```python
from build123d import *

# Parameters (mm, degrees)
SKETCH1_W                = 2
SKETCH1_H                = 6
BOSS_EXTRUDE1_DEPTH      = 8
BOSS_EXTRUDE1_2_DEPTH    = 8
BOSS_EXTRUDE2_DEPTH      = 6
FILLET2_R                = 3
SKETCH3_R                = 1.65
CUT_EXTRUDE1_DEPTH       = 90.043007931
FILLET3_R                = 6
CIRPATTERN2_COUNT        = 3
FILLET2_OF_CIRPATTERN2_R = 3
FILLET3_OF_CIRPATTERN2_R = 6
SKETCH4_R                = 2
CUT_EXTRUDE2_DEPTH       = 80.425963387
CHAMFER1_SIZE            = 1


with BuildPart() as part:
    # Sketch1 → Boss-Extrude1 (new body)
    with BuildSketch(Plane(origin=(0, 0, 0), x_dir=(1, 0, 0), z_dir=(0, 1, 0))):
        with Locations((-24, 50)):
            Rectangle(SKETCH1_W, SKETCH1_H)
    boss_extrude1 = extrude(amount=BOSS_EXTRUDE1_DEPTH)



with BuildPart() as body_2:
    # Sketch1 → Boss-Extrude1 2 (new body)
    with BuildSketch(Plane(origin=(0, 0, 0), x_dir=(1, 0, 0), z_dir=(0, 1, 0))):
        with Locations((24, 50)):
            Rectangle(SKETCH1_W, SKETCH1_H)
    boss_extrude1_2 = extrude(amount=BOSS_EXTRUDE1_2_DEPTH)


with BuildPart() as part_1:
    add(part.part)

    add(body_2.part)  # Boss-Extrude2 merges body 2
    # Sketch2 → Boss-Extrude2 (add)
    with BuildSketch(Plane(origin=(0, 0, 0), x_dir=(1, 0, 0), z_dir=(0, 1, 0))):
        with BuildLine():
            Line((25, 53), (-25, 53))
            Line((-25, 53), (-25, 47))
            ThreePointArc((-25, 47), (-36.983431799, 38.291327639), (-46.103145229, 26.617663308))
            Line((-46.103145229, 26.617663308), (-36.806079661, 21.25))
            ThreePointArc((-36.806079661, 21.25), (0, 42.5), (36.806079661, 21.25))
            Line((36.806079661, 21.25), (46.103145229, 26.617663308))
            ThreePointArc((46.103145229, 26.617663308), (36.983431799, 38.291327639), (25, 47))
            Line((25, 47), (25, 53))
        make_face()
    boss_extrude2 = extrude(amount=-BOSS_EXTRUDE2_DEPTH)

    # Fillet2
    fillet2_edges = [part_1.edges().sort_by_distance(p)[0] for p in [
        (24, 8, -47),
        (24, 8, -53),
        (-24, 8, -47),
        (-24, 8, -53),
    ]]
    fillet(fillet2_edges, radius=FILLET2_R - 0.0001)  # a hair under: the kernel refuses the full size

    # Sketch3 → Cut-Extrude1 (cut, through all)
    with BuildSketch(Plane(origin=(25, 0, 0), x_dir=(0, 0, -1), z_dir=(1, 0, 0))):
        with Locations((50, 5)):
            Circle(SKETCH3_R)
    cut_extrude1 = extrude(amount=-CUT_EXTRUDE1_DEPTH, mode=Mode.SUBTRACT)

    # Fillet3
    fillet3_edges = [part_1.edges().sort_by_distance(p)[0] for p in [
        (0, -6, -53),
    ]]
    fillet(fillet3_edges, radius=FILLET3_R - 0.0001)  # a hair under: the kernel refuses the full size

    # CirPattern2: Boss-Extrude1, Boss-Extrude1 2, Boss-Extrude2, Cut-Extrude1 ×3 about axis
    cirpattern2_axis = Axis((0, 0, 0), (0, 1, 0))
    add([boss_extrude1.rotate(cirpattern2_axis, i * 360 / CIRPATTERN2_COUNT) for i in range(1, CIRPATTERN2_COUNT)])
    add([boss_extrude1_2.rotate(cirpattern2_axis, i * 360 / CIRPATTERN2_COUNT) for i in range(1, CIRPATTERN2_COUNT)])
    add([boss_extrude2.rotate(cirpattern2_axis, i * 360 / CIRPATTERN2_COUNT) for i in range(1, CIRPATTERN2_COUNT)])
    add([cut_extrude1.rotate(cirpattern2_axis, i * 360 / CIRPATTERN2_COUNT) for i in range(1, CIRPATTERN2_COUNT)], mode=Mode.SUBTRACT)

    # Fillet2 of CirPattern2
    fillet2_of_cirpattern2_edges = [part_1.edges().sort_by_distance(p)[0] for p in [
        (-52.703193978, 8, 2.715390309),
        (-57.899346401, 8, 5.715390309),
        (-28.703193978, 8, 44.284609691),
        (-33.899346401, 8, 47.284609691),
        (28.703193978, 8, 44.284609691),
        (33.899346401, 8, 47.284609691),
        (52.703193978, 8, 2.715390309),
        (57.899346401, 8, 5.715390309),
    ]]
    fillet(fillet2_of_cirpattern2_edges, radius=FILLET2_OF_CIRPATTERN2_R - 0.0001)  # a hair under: the kernel refuses the full size

    # Fillet3 of CirPattern2
    fillet3_of_cirpattern2_edges = [part_1.edges().sort_by_distance(p)[0] for p in [
        (-45.899346401, -6, 26.5),
        (45.899346401, -6, 26.5),
    ]]
    fillet(fillet3_of_cirpattern2_edges, radius=FILLET3_OF_CIRPATTERN2_R - 0.0001)  # a hair under: the kernel refuses the full size

    # Sketch4 → Cut-Extrude2 (cut, through all)
    with BuildSketch(Plane(origin=(0, 0, 0), x_dir=(1, 0, 0), z_dir=(0, 1, 0))):
        with Locations(Location((-41.13620668, 23.75, 0), (0, 0, 270))):
            Circle(SKETCH4_R)
        with Locations(Location((-24.052579046, 40.960022476, 0), (0, 0, 270))):
            Circle(SKETCH4_R)
        with Locations(Location((-47.498709527, 0.350133242, 0), (0, 0, 270))):
            Circle(SKETCH4_R)
        with Locations(Location((-33.711135616, 33.463552344, 0), (0, 0, 270))):
            Circle(SKETCH4_R)
        with Locations(Location((-45.835854239, 12.462923661, 0), (0, 0, 270))):
            Circle(SKETCH4_R)
        with Locations(Location((47.498709527, 0.350133242, 0), (0, 0, 270))):
            Circle(SKETCH4_R)
        with Locations(Location((45.835854239, 12.462923661, 0), (0, 0, 270))):
            Circle(SKETCH4_R)
        with Locations(Location((41.13620668, 23.75, 0), (0, 0, 270))):
            Circle(SKETCH4_R)
        with Locations(Location((33.711135616, 33.463552344, 0), (0, 0, 270))):
            Circle(SKETCH4_R)
        with Locations(Location((24.052579046, 40.960022476, 0), (0, 0, 270))):
            Circle(SKETCH4_R)
        with Locations(Location((-23.446130481, -41.310155718, 0), (0, 0, 270))):
            Circle(SKETCH4_R)
        with Locations(Location((-12.124718623, -45.926476006, 0), (0, 0, 270))):
            Circle(SKETCH4_R)
        with Locations(Location((0, -47.5, 0), (0, 0, 270))):
            Circle(SKETCH4_R)
        with Locations(Location((12.124718623, -45.926476006, 0), (0, 0, 270))):
            Circle(SKETCH4_R)
        with Locations(Location((23.446130481, -41.310155718, 0), (0, 0, 270))):
            Circle(SKETCH4_R)
    extrude(amount=-CUT_EXTRUDE2_DEPTH, mode=Mode.SUBTRACT)

    # Chamfer1
    chamfer1_edges = [part_1.edges().sort_by_distance(p)[0] for p in [
        (-41.13620668, 0, -25.75),
        (-24.052579046, 0, -42.960022476),
        (-47.498709527, 0, -2.350133242),
        (-33.711135616, 0, -35.463552344),
        (-45.835854239, 0, -14.462923661),
        (41.13620668, 0, -25.75),
        (47.498709527, 0, -2.350133242),
        (24.052579046, 0, -42.960022476),
        (45.835854239, 0, -14.462923661),
        (33.711135616, 0, -35.463552344),
        (0, 0, 45.5),
        (-23.446130481, 0, 39.310155718),
        (23.446130481, 0, 39.310155718),
        (-12.124718623, 0, 43.926476006),
        (12.124718623, 0, 43.926476006),
    ]]
    chamfer(chamfer1_edges, length=CHAMFER1_SIZE)


solid = part_1.part
```
Design review of the part built by this model. Coordinates are the model's own, in mm. A direction names the side the tool comes from. Coordinates: 2 decimals unless noted, no trailing zeros. Write each loop counter-clockwise with the first axis right and the second up, starting at its lowest first coordinate (ties: lowest second). Pieces come first, ordered by that corner, then holes. Notation, with made-up numbers: M -27.75,-13.5 L -13.75,-13.5 A24 cw -13.75,22.5 Z; hole C 14,51 d4. An arc over 180 degrees is marked long. Answer as a JSON object with one key per item and string values.
Item 1: Draft analysis for pull direction Y (two halves, no side actions). For faces 4 (the flat face through (30.765, 1.098, 46.63)), 5 (the cylindrical face through (-53.88, 5.07, 3.38)), 6 (the cylindrical face through (53.437, 7.098, 3.155)), state which applies: pulls with the +Y half, pulls with the -Y half, needs draft (parallel to the pull), parting line crosses it, or undercut.
Outcome:
{"face 4": "needs draft", "face 5": "undercut", "face 6": "pulls with the +Y half"}
Item 2: Add section B-B, the plane z = -23.75. Give the boundary of the cut face in (x, y).
Outcome:
{"outline": "M -47.64,-6 L -43.14,-6 L -43.14,-1 L -44.14,0 L -47.64,0 Z; M -39.14,-6 L -35.24,-6 L -35.24,0 L -38.14,0 L -39.14,-1 Z; M 35.24,-6 L 39.14,-6 L 39.14,-1 L 38.14,0 L 35.24,0 Z; M 43.14,-6 L 47.64,-6 L 47.64,0 L 44.14,0 L 43.14,-1 Z"}
Item 3: Machinability: for faces 1 (the flat face through (-30.838, 1.098, 46.672)), 2 (the cylindrical face through (35.1, -3.5, -34.9)), 3 (the cylindrical face through (29.44, 7.1, 44.72)), which of the approach directions +Z, -Z, +X, -X, +Y, -Y give a long, thin tool a straight path to every point of the face, cutting with its end or side? Answer none if there is none.
Outcome:
{"face 1": "+Z, +Y, -Y", "face 2": "+Y, -Y", "face 3": "-Z, +Y"}
Item 4: Wall thickness on probe 1 along X at (y, z) = (-3, -12); probe 2 along X at (y, z) = (-3.5, 1); probe 3 along Y at (x, z) = (-46.5, 8): over which ranges is each line inside the solid? List them lowest first.
Outcome:
{"probe 1": "-51.87 to -47.78, -43.89 to -40.77, 40.77 to 43.89, 47.78 to 51.87", "probe 2": "-53.23 to -48.97, -46.02 to -42.49, 42.49 to 46.02, 48.97 to 53.23", "probe 3": "-6 to 0"}
Item 5: Add section A-A, the plane y = 2. Give the boundary of the cut face in (x, z).
Outcome:
{"outline": "M -58.4,4.85 L -53.2,1.85 L -52.2,3.58 L -57.4,6.58 Z; M -34.4,46.42 L -29.2,43.42 L -28.2,45.15 L -33.4,48.15 Z; M -25,-53 L -23,-53 L -23,-47 L -25,-47 Z; M 23,-53 L 25,-53 L 25,-47 L 23,-47 Z; M 28.2,45.15 L 29.2,43.42 L 34.4,46.42 L 33.4,48.15 Z; M 52.2,3.58 L 53.2,1.85 L 58.4,4.85 L 57.4,6.58 Z"}
Item 6: Insertion check: pin 1 Ø5 at (x, z) = (-41.14, -23.75) entering from -Y; pin 2 Ø1.8 at (y, z) = (3.5, -51.5) entering from -X; pin 3 Ø6 at (y, z) = (-3, 24) entering from +X; pin 4 Ø4.5 at (x, z) = (-47.5, -0.35) entering from +Y. Each pin has a flat end and moves straight along its axis. Give the tip position at first contact, or say it passes through.
Outcome:
{"pin 1": "y = -6", "pin 2": "x = -25", "pin 3": "x = 48.62", "pin 4": "y = -0.75"}
